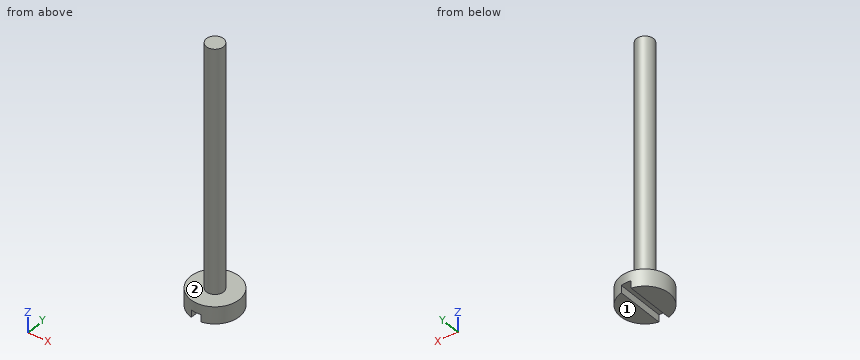
```python
from build123d import *

# Parameters (mm, degrees)
SKETCH1_R           = 1
BOSS_EXTRUDE1_DEPTH = 0.7
SKETCH3_R           = 0.35
BOSS_EXTRUDE2_DEPTH = 10
SKETCH5_W           = 0.4
SKETCH5_H           = 2
CUT_EXTRUDE1_DEPTH  = 0.3


with BuildPart() as part:
    # Sketch1 → Boss-Extrude1 (new body)
    with BuildSketch(Plane.XY):
        Circle(SKETCH1_R)
    extrude(amount=BOSS_EXTRUDE1_DEPTH)

    # Sketch3 → Boss-Extrude2 (add)
    with BuildSketch(Plane.XY.offset(0.7)):
        Circle(SKETCH3_R)
    extrude(amount=BOSS_EXTRUDE2_DEPTH)

    # Sketch5 → Cut-Extrude1 (cut)
    with BuildSketch(Plane(origin=(0, 0, 0), x_dir=(-1, 0, 0), z_dir=(0, 0, -1))):
        Rectangle(SKETCH5_W, SKETCH5_H)
    extrude(amount=-CUT_EXTRUDE1_DEPTH, mode=Mode.SUBTRACT)


solid = part.part
```
Input: part model. Units: mm. Frame: model coordinates. Face numbers are marked on the shaded views. A direction names the side the tool comes from. Give positions to 0.01 mm unless a question says otherwise; leave off trailing zeros. Write each loop counter-clockwise with the first axis right and the second up, starting at its lowest first coordinate (ties: lowest second). Pieces come first, ordered by that corner, then holes. Notation, with made-up numbers: (-21, 2) - (-10, 2) arc R15 ccw to (-10, 30) - close; hole circle Ø8 at (39.25, -6.5). An arc over 180 degrees is marked (long way). Write item = value, one per line. Start each with the question number.
1) Cut plane C-C (z = 9). Return loops of the section in (x, y).
2) Cut plane B-B (y = 0). Return loops of the section in (x, z).
3) Cut plane A-A (x = 0). Return loops of the section in (y, z), and give its area (3 significant figures).
4) Reachability of the marked faces 1 and 2 from +Z, -Z, +X, -X, +Y, -Y: full face, straight path, thin tool, end or side. Return the list, or none.
5) Cut plane D-D (y = 0.7). Return loops of the section in (x, z).
6) Material intervals for L1, parallel to Z at x = 0.7, y = 0.65; L2, parallel to Z at x = 0.15, y = -0.45; L3, parallel to Y at x = -0.1, z = 8.5, sorted ascending. Write a range as [from, to].
Answers follow:
q1.outline = circle Ø0.7 at (0, 0)
q2.outline = (-1, 0) - (-0.2, 0) - (-0.2, 0.3) - (0.2, 0.3) - (0.2, 0) - (1, 0) - (1, 0.7) - (0.35, 0.7) - (0.35, 10.7) - (-0.35, 10.7) - (-0.35, 0.7) - (-1, 0.7) - close
q3.outline = (-1, 0.3) - (1, 0.3) - (1, 0.7) - (0.35, 0.7) - (0.35, 10.7) - (-0.35, 10.7) - (-0.35, 0.7) - (-1, 0.7) - close
q3.area = 7.80 mm^2
q4.face_1 = -Z, +X, -X, +Y, -Y
q4.face_2 = +Z
q5.outline = (-0.71, 0) - (-0.2, 0) - (-0.2, 0.3) - (0.2, 0.3) - (0.2, 0) - (0.71, 0) - (0.71, 0.7) - (-0.71, 0.7) - close
q6.L1 = [0, 0.7]
q6.L2 = [0.3, 0.7]
q6.L3 = [-0.34, 0.34]
